```python
from build123d import *

# Parameters (mm, degrees)
SALIENTE_EXTRUIR1_DEPTH = 30
CORTAR_EXTRUIR1_DEPTH   = 3
CROQUIS3_R              = 1.5
CORTAR_EXTRUIR2_DEPTH   = 3


with BuildPart() as part:
    # Croquis1 → Saliente-Extruir1 (new body)
    with BuildSketch(Plane.XY):
        Polygon((-64.928571429, 65.135714286), (-64.928571429, 62.135714286), (-4.928571429, 62.135714286), (-4.928571429, -7.864285714), (-1.928571429, -7.864285714), (-1.928571429, 65.135714286), align=None)
    extrude(amount=SALIENTE_EXTRUIR1_DEPTH)

    # Croquis2 → Cortar-Extruir1 (cut)
    with BuildSketch(Plane(origin=(0, 65.135714286, 0), x_dir=(1, 0, 0), z_dir=(0, 1, 0))):
        with BuildLine():
            Line((-59.928571429, -24.5), (-44.928571429, -24.5))
            ThreePointArc((-44.928571429, -24.5), (-43.428571429, -23), (-44.928571429, -21.5))
            Line((-44.928571429, -21.5), (-59.928571429, -21.5))
            ThreePointArc((-59.928571429, -21.5), (-61.428571429, -23), (-59.928571429, -24.5))
        make_face()
        with BuildLine():
            Line((-59.928571429, -8.5), (-44.928571429, -8.5))
            ThreePointArc((-44.928571429, -8.5), (-43.428571429, -7), (-44.928571429, -5.5))
            Line((-44.928571429, -5.5), (-59.928571429, -5.5))
            ThreePointArc((-59.928571429, -5.5), (-61.428571429, -7), (-59.928571429, -8.5))
        make_face()
    extrude(amount=-CORTAR_EXTRUIR1_DEPTH, mode=Mode.SUBTRACT)

    # Croquis3 → Cortar-Extruir2 (cut)
    with BuildSketch(Plane.ZY.offset(4.928571429)):
        with Locations(Location((20.656854249, 1.478860036, 0), (0, 0, 270))):
            Circle(CROQUIS3_R)
        with Locations(Location((9.343145751, 1.478860036, 0), (0, 0, 270))):
            Circle(CROQUIS3_R)
        with Locations(Location((9.343145751, 12.792568535, 0), (0, 0, 270))):
            Circle(CROQUIS3_R)
        with Locations(Location((20.656854249, 12.792568535, 0), (0, 0, 270))):
            Circle(CROQUIS3_R)
    extrude(amount=-CORTAR_EXTRUIR2_DEPTH, mode=Mode.SUBTRACT)


solid = part.part
```
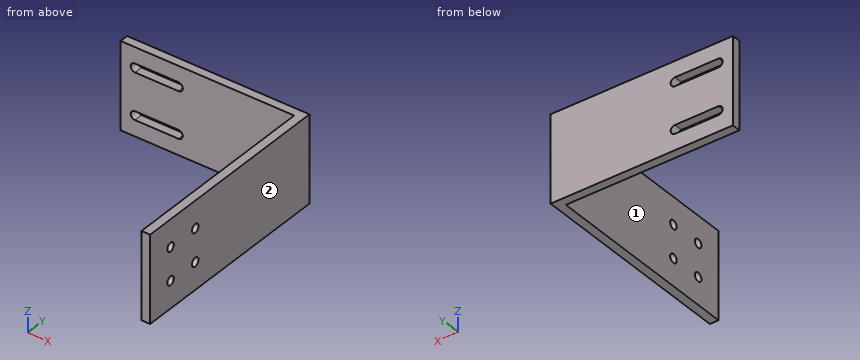
Can you work these out from the model? Positions are in its coordinate system, mm. Face numbers are marked on the shaded views. A direction names the side the tool comes from. Round coordinates to 2 decimals unless told otherwise and drop trailing zeros. Loops run counter-clockwise (first coordinate to the right, second up) from the corner with the lowest first, then second, coordinate; pieces in that order, holes last. Notation, with made-up numbers: (44.5, 6) -> (53.5, 6) arc R21 ccw to (53.5, 26) -> close; hole circle Ø9 at (83.25, 18.5). An arc over 180 degrees is marked (long way). Answer in a Markdown table with one row per item.
Item 1: Suppose I cut it at C-C, the plane y = 43. List the corners of the cut face in (x, z) for me.
Answer block:
| item | result |
|---|---|
| outline | (-4.93, 0) -> (-1.93, 0) -> (-1.93, 30) -> (-4.93, 30) -> close |
Item 2: If I drill on probe 1 along Y at (x, z) = (-30, 27.75); probe 2 along X at (y, z) = (38, 22), over which ranges is the centre line in solid material (lowest first)?
Answer block:
| item | result |
|---|---|
| probe 1 | 62.14 to 65.14 |
| probe 2 | -4.93 to -1.93 |
Item 3: On a 3-axis mill with a long thin cutter (end or side, diameter ignored), from which of +Z, -Z, +X, -X, +Y, -Y can I reach the whole of each face in a straight line? I mean the marked faces 1 and 2. Say none if no direction works.
Answer block:
| item | result |
|---|---|
| face 1 | +Z, -Z, -X, -Y |
| face 2 | +Z, -Z, +X, +Y, -Y |
Item 4: Will these pins go through, and if not, where does the flat tip stop? P1, Ø3.5, axis at y = 1.48, z = 20.66, coming from the +X side; P2, Ø6, axis at y = 30, z = 15, coming from the -X side; P3, Ø8, axis at x = -45, z = 18, coming from the -Y side.
Answer block:
| item | result |
|---|---|
| P1 | x = -1.93 |
| P2 | x = -4.93 |
| P3 | y = 62.14 |
Item 5: Suppose I cut it at B-B, the plane x = -48. List the corners of the cut face in (y, z) for me, plus the area to 3 significant figures.
Answer block:
| item | result |
|---|---|
| outline | (62.14, 0) -> (65.14, 0) -> (65.14, 5.5) -> (62.14, 5.5) -> close; (62.14, 8.5) -> (65.14, 8.5) -> (65.14, 21.5) -> (62.14, 21.5) -> close; (62.14, 24.5) -> (65.14, 24.5) -> (65.14, 30) -> (62.14, 30) -> close |
| area | 72.0 mm² |
Item 6: Suppose I cut it at D-D, the plane z = 23.5. List the corners of the cut face in (x, y) for me, plus the area to 3 significant figures.
Answer block:
| item | result |
|---|---|
| outline | (-64.93, 62.14) -> (-61.34, 62.14) -> (-61.34, 65.14) -> (-64.93, 65.14) -> close; (-43.51, 62.14) -> (-4.93, 62.14) -> (-4.93, -7.86) -> (-1.93, -7.86) -> (-1.93, 65.14) -> (-43.51, 65.14) -> close |
| area | 346 mm² |
Item 7: Suppose I cut it at A-A, the plane z = 7. List the corners of the cut face in (x, y) for me, plus the area to 3 significant figures.
Answer block:
| item | result |
|---|---|
| outline | (-64.93, 62.14) -> (-61.43, 62.14) -> (-61.43, 65.14) -> (-64.93, 65.14) -> close; (-43.43, 62.14) -> (-4.93, 62.14) -> (-4.93, -7.86) -> (-1.93, -7.86) -> (-1.93, 65.14) -> (-43.43, 65.14) -> close |
| area | 345 mm² |
